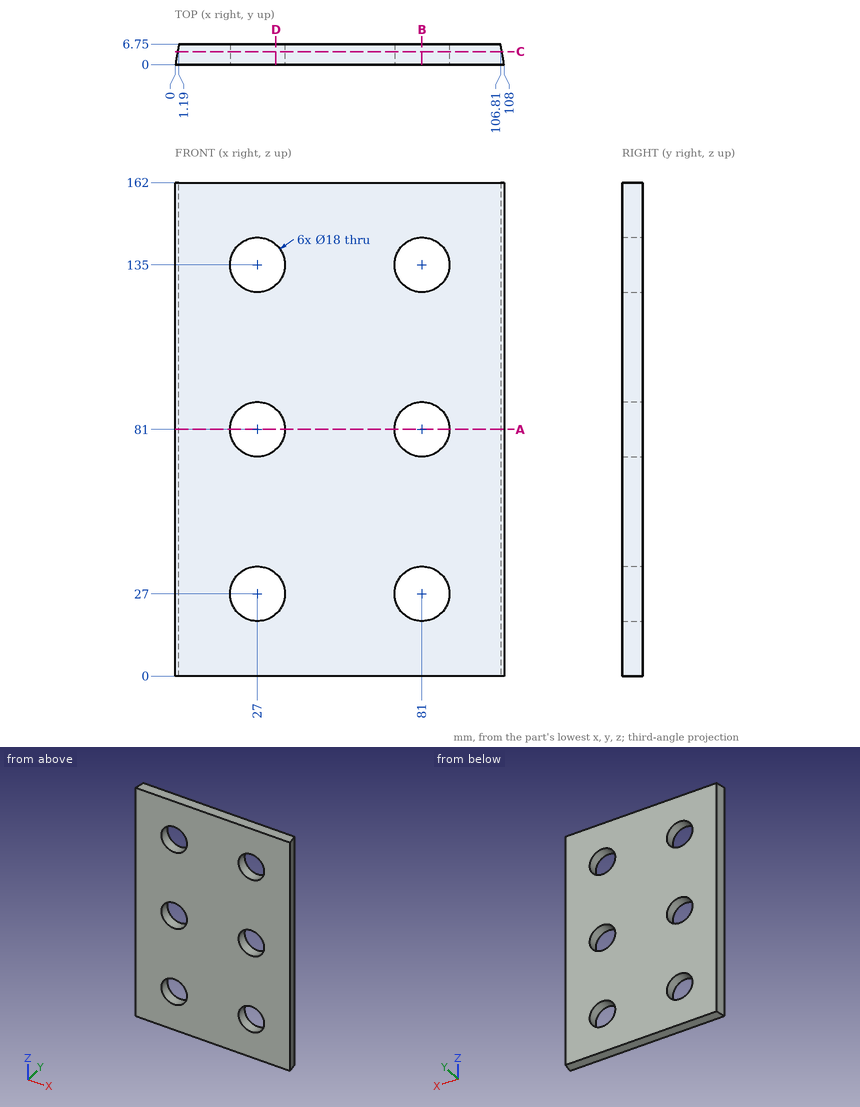
Design review of the part shown in the three views and the two pictorial views. Dimensions are in mm from the part's minimum x, y and z. Round coordinates to 2 decimals unless told otherwise and drop trailing zeros. Order: outer loops, then holes, each group sorted by start corner. A loop starts at its lowest first (then second) coordinate and runs counter-clockwise, first axis right, second up.
(1) Wall thickness on L1, parallel to X at y = 5, z = 135; L2, parallel to X at y = 1.75, z = 27; L3, parallel to Z at x = 84, y = 2 (1 decimal): over which ranges is each line inside the solid? List them lowest first.
Working result:
L1: x = 0.88 to 18, 36 to 72, 90 to 107.12
L2: x = 0.31 to 18, 36 to 72, 90 to 107.69
L3: z = 0 to 18.5, 35.5 to 72.5, 89.5 to 126.5, 143.5 to 162
(2) Take a section at A-A, the plane z = 81. Count the separate pieces of the cut face and the enclosed holes in it, plus the area to 3 significant figures.
Working result:
separate pieces: 3
enclosed holes: 0
area: 478 mm2
(3) Take a section at B-B, the plane x = 81. State the section outline as (y, z) points, plus the area to 3 significant figures.
Working result:
outline: (0, 0) - (6.75, 0) - (6.75, 18) - (0, 18) - close; (0, 36) - (6.75, 36) - (6.75, 72) - (0, 72) - close; (0, 90) - (6.75, 90) - (6.75, 126) - (0, 126) - close; (0, 144) - (6.75, 144) - (6.75, 162) - (0, 162) - close
area: 729 mm2
(4) Take a section at C-C, the plane y = 4.25. State the section outline as (x, z) points.
Working result:
outline: (0.75, 0) - (107.25, 0) - (107.25, 162) - (0.75, 162) - close; hole circle Ø18 at (27, 27); hole circle Ø18 at (27, 81); hole circle Ø18 at (27, 135); hole circle Ø18 at (81, 27); hole circle Ø18 at (81, 81); hole circle Ø18 at (81, 135)
(5) Take a section at D-D, the plane x = 33. State the section outline as (y, z) points, plus the area to 3 significant figures.
Working result:
outline: (0, 0) - (6.75, 0) - (6.75, 20.29) - (0, 20.29) - close; (0, 33.71) - (6.75, 33.71) - (6.75, 74.29) - (0, 74.29) - close; (0, 87.71) - (6.75, 87.71) - (6.75, 128.29) - (0, 128.29) - close; (0, 141.71) - (6.75, 141.71) - (6.75, 162) - (0, 162) - close
area: 822 mm2
